```python
from build123d import *

# Parameters (mm, degrees)
SKETCH1_R           = 4
SKETCH1_R_2         = 1.85
BOSS_EXTRUDE1_DEPTH = 12.5
FILLET1_R           = 10
FILLET2_R           = 3
FILLET3_R           = 10
CUT_EXTRUDE1_DEPTH  = 20


with BuildPart() as part:
    # Sketch1 → Boss-Extrude1 (new body)
    with BuildSketch(Plane.XY):
        with BuildLine():
            Line((14.142135624, 14.142135624), (28.284271247, 28.284271247))
            ThreePointArc((28.284271247, 28.284271247), (-6.945927107, 39.39231012), (-36.252311481, 16.90473047))
            Line((-36.252311481, 16.90473047), (-45.315389352, 21.130913087))
            ThreePointArc((-45.315389352, 21.130913087), (46.768835106, 17.682648638), (-20, -45.82575695))
            Line((-20, -45.82575695), (-20, 0))
            ThreePointArc((-20, 0), (-7.653668647, 18.47759065), (14.142135624, 14.142135624))
        make_face()
        Circle(SKETCH1_R, mode=Mode.SUBTRACT)
        with Locations((0, 8)):
            Circle(SKETCH1_R_2, mode=Mode.SUBTRACT)
        with Locations((8, 0)):
            Circle(SKETCH1_R_2, mode=Mode.SUBTRACT)
        with Locations((0, -8)):
            Circle(SKETCH1_R_2, mode=Mode.SUBTRACT)
        with Locations((-8, 0)):
            Circle(SKETCH1_R_2, mode=Mode.SUBTRACT)
    extrude(amount=BOSS_EXTRUDE1_DEPTH)

    # Fillet1
    fillet1_edges = [part.edges().sort_by_distance(p)[0] for p in [
        (28.284271247, 28.284271247, 6.25),
        (14.142135624, 14.142135624, 6.25),
    ]]
    fillet(fillet1_edges, radius=FILLET1_R - 0.0001)  # a hair under: the kernel refuses the full size

    # Fillet2
    fillet2_edges = [part.edges().sort_by_distance(p)[0] for p in [
        (-36.252311481, 16.90473047, 6.25),
        (-45.315389352, 21.130913087, 6.25),
    ]]
    fillet(fillet2_edges, radius=FILLET2_R)

    # Fillet3
    fillet3_edges = [part.edges().sort_by_distance(p)[0] for p in [
        (-20, -45.82575695, 6.25),
    ]]
    fillet(fillet3_edges, radius=FILLET3_R)

    # Sketch3 → Cut-Extrude1 (cut)
    with BuildSketch(Plane(origin=(0, 0, 0), x_dir=(0, -1, 0), z_dir=(-0.1564344650402244, 0, -0.9876883405951388))):
        Polygon((-59.412445721, 3.059679317), (-37.456599692, -8.541700414), (-10.399971435, 42.663516366), (-32.355817465, 54.264896097), align=None)
    extrude(amount=CUT_EXTRUDE1_DEPTH, mode=Mode.SUBTRACT)


solid = part.part
```
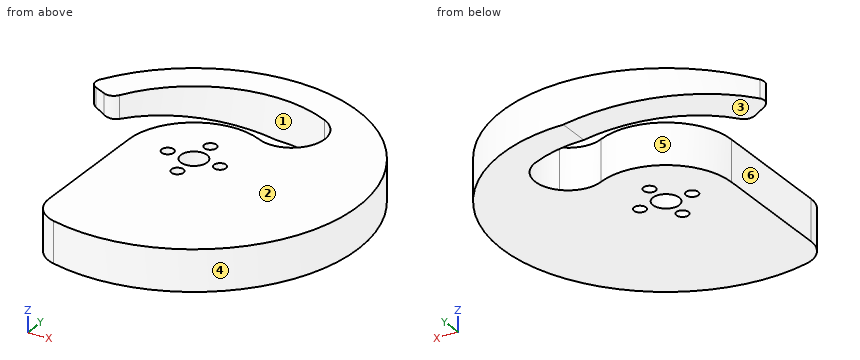
Input: part model. Units: mm. Frame: model coordinates. Face numbers are marked on the shaded views. A direction names the side the tool comes from. Give positions to 0.01 mm unless a question says otherwise; leave off trailing zeros. Order: outer loops, then holes, each group sorted by start corner. A loop starts at its lowest first (then second) coordinate and runs counter-clockwise, first axis right, second up. Notation, with made-up numbers: M -19.5,86.25 L 9.5,86.25 A20 cw 9.5,112.25 Z; hole C 28.25,-10 d3. An arc over 180 degrees is marked long. Return JSON: item names as keys, results as strings.
Item 1: Cut plane D-D (y = -12). Return loops of the section in (x, z), then the cut area to 3 significant figures.
Solutions:
{"outline": "M -20,0 L 48.54,0 L 48.54,12.5 L -20,12.5 Z", "area": "857 mm^2"}
Item 2: Cut plane C-C (x = 32). Return loops of the section in (y, z).
Solutions:
{"outline": "M -38.42,0 L 38.42,0 L 38.42,12.5 L -38.42,12.5 Z"}
Item 3: Access query for the marked faces 1, 2 and 3. Directions: +Z, -Z, +X, -X, +Y, -Y. A direction counts if a zero-diameter tool reaches every point of the face in a straight line with its end or side. Return the directions, or none.
Solutions:
{"face 1": "+Z, -Z", "face 2": "+Z, +X, -X, +Y, -Y", "face 3": "-Z, -X, +Y"}
Item 4: Cut plane A-A (z = 3.75). State how many separate pieces and enclosed holes the cut face has, then the cut area to 3 significant figures.
Solutions:
{"separate pieces": "1", "enclosed holes": "5", "area": "4,940 mm^2"}
Item 5: Pull-direction query (Y, two-part tool) for the marked faces 4, 5 and 6; classes: +Y half, -Y half, draft (parallel to the pull), parting line (faces both ways), or undercut.
Solutions:
{"face 4": "parting line", "face 5": "undercut", "face 6": "draft"}
Item 6: First-contact query: P1, Ø1.5, axis at x = 8, y = 16.5, coming from the -Z side; P2, Ø6, axis at x = -4, z = 5, coming from the +Y side; P3, Ø4, axis at y = -10.5, z = 6, coming from the -X side. Flat tips, straight axial feed; report the tip coordinate or a pass-through.
Solutions:
{"P1": "z = 0", "P2": "y = 49.99", "P3": "x = -20"}
Item 7: Cut plane B-B (y = 8). Return loops of the section in (x, z), then the cut area to 3 significant figures.
Solutions:
{"outline": "M -18.33,0 L -1.85,0 L -1.85,12.5 L -18.33,12.5 Z; M 1.85,0 L 49.36,0 L 49.36,12.5 L 1.85,12.5 Z", "area": "800 mm^2"}
Item 8: Ray query, probe 1 along Y at (x, z) = (0, 9); probe 2 along Y at (x, z) = (8, 8.75); probe 3 along X at (y, z) = (0.5, 5.5). Return the intervals inside material, ascending.
Solutions:
{"probe 1": "-50 to -9.85, -6.15 to -4, 4 to 6.15, 9.85 to 20, 40 to 50", "probe 2": "-49.36 to -1.85, 1.85 to 18.33, 39.19 to 49.36", "probe 3": "-19.99 to -9.78, -6.22 to -3.97, 3.97 to 6.22, 9.78 to 50"}
